```python
from build123d import *

# Parameters (mm, degrees)
SKETCH1_W           = 736.6
SKETCH1_H           = 381
BOSS_EXTRUDE1_DEPTH = 76.2
SKETCH2_W           = 50.8
SKETCH2_H           = 76.2
BOSS_EXTRUDE2_DEPTH = 254
SKETCH3_R           = 12.7
CUT_EXTRUDE1_DEPTH  = 503.413027299
SHELL1_T            = -2.54
SKETCH4_R           = 184.15
CUT_EXTRUDE2_DEPTH  = 2.54
SKETCH5_R           = 6.621401099
CUT_EXTRUDE3_DEPTH  = 1219.2


with BuildPart() as part:
    # Sketch1 → Boss-Extrude1 (new body)
    with BuildSketch(Plane(origin=(0, 0, 0), x_dir=(1, 0, 0), z_dir=(0, 1, 0))):
        Rectangle(SKETCH1_W, SKETCH1_H)
    extrude(amount=BOSS_EXTRUDE1_DEPTH)

    # Sketch2 → Boss-Extrude2 (add)
    with BuildSketch(Plane(origin=(0, 0, 0), x_dir=(-1, 0, 0), z_dir=(0, -1, 0))):
        with Locations((-317.5, 0)):
            Rectangle(SKETCH2_W, SKETCH2_H)
    extrude(amount=BOSS_EXTRUDE2_DEPTH)

    # Sketch3 → Cut-Extrude1 (cut, through all)
    with BuildSketch(Plane.XY.offset(38.1)):
        with Locations((317.5, -228.6)):
            Circle(SKETCH3_R)
    extrude(amount=-CUT_EXTRUDE1_DEPTH, mode=Mode.SUBTRACT)

    # Shell1
    shell1_openings = [part.faces().sort_by_distance(p)[0] for p in [
        (-368.3, 38.1, 0),
        (368.3, 38.1, 0),
    ]]
    offset(amount=SHELL1_T, openings=shell1_openings, kind=Kind.INTERSECTION)

    # Sketch4 → Cut-Extrude2 (cut)
    with BuildSketch(Plane(origin=(0, 76.2, 0), x_dir=(1, 0, 0), z_dir=(0, 1, 0))):
        with Locations(Location((-63.5, 0, 0), (0, 0, 270))):
            Circle(SKETCH4_R)
    extrude(amount=-CUT_EXTRUDE2_DEPTH, mode=Mode.SUBTRACT)

    # Sketch5 → Cut-Extrude3 (cut)
    with BuildSketch(Plane(origin=(0, 76.2, 0), x_dir=(1, 0, 0), z_dir=(0, 1, 0))):
        with Locations(Location((-63.5, 0, 0), (0, 0, 270))):
            Circle(SKETCH5_R)
    extrude(amount=-CUT_EXTRUDE3_DEPTH, mode=Mode.SUBTRACT)


solid = part.part
```
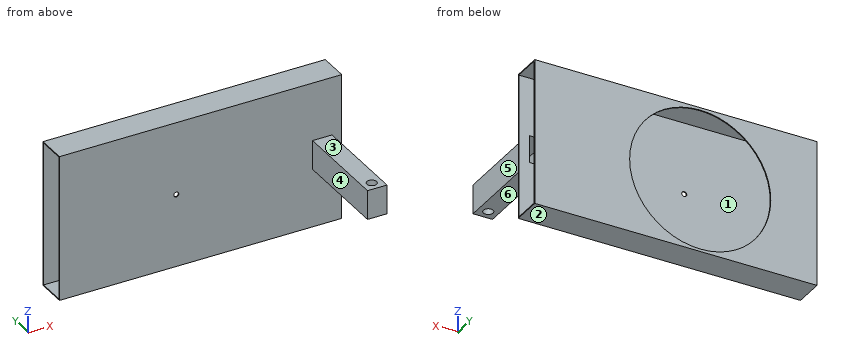
Geometry check sheet. Reference: the model listing, model coordinates, mm. Face numbers are marked on the shaded views. A direction names the side the tool comes from. Coordinates: 2 decimals unless noted, no trailing zeros. Order: outer loops, then holes, each group sorted by start corner. A loop starts at its lowest first (then second) coordinate and runs counter-clockwise, first axis right, second up. Notation, with made-up numbers: (82, -17.5) - (100, -17.5) arc R26 ccw to (100, 0.5) - close; hole circle Ø7 at (4, -2). An arc over 180 degrees is marked (long way). Answer in a Markdown table with one row per item. Add a question column.
1. Section check C-C (x = 168.5). Enter the section's corners in (y, z).
2. Access from +Z, -Z, +X, -X, +Y, -Y to the whole of each face (thin tool, end or side, straight path). Record for the marked faces 1, 2 and 3.
3. Section check B-B (x = 317.5). Enter the section's corners in (y, z), plus the area to 3 significant figures.
4. Material ranges on L1, parallel to X at y = 1, z = 0; L2, parallel to Y at x = 317, z = 21; L3, parallel to Y at x = -210.5, z = -165, recorded low to high. Write a range as [from, to].
5. Section check A-A (y = 13). Enter the section's corners in (x, z).
6. Section check D-D (y = -32.5). Enter the section's corners in (x, z).
7. Gauge pin test, flat ends, axial feed: pin 1 Ø1.5 at (x, z) = (136, 3.5) entering from -Y; pin 2 Ø23 at (x, y) = (307, -167) entering from +Z. Record the tip position at first contact, or that the pin passes through.
8. Draft check along X on the marked faces 4, 5 and 6. Enter one of: +X half, -X half, draft (parallel to the pull), parting line (faces both ways), or undercut.
Data:
| question | item | result |
|---|---|---|
| 1 | outline | (0, -190.5) - (76.2, -190.5) - (76.2, 190.5) - (0, 190.5) - close; hole (2.54, -187.96) - (73.66, -187.96) - (73.66, 187.96) - (2.54, 187.96) - close |
| 2 | face 1 | +X, -X |
| 2 | face 2 | -Z, +X, -X, +Y, -Y |
| 2 | face 3 | +Z, +X, -X, -Y |
| 3 | outline | (-254, -38.1) - (-241.3, -38.1) - (-241.3, 38.1) - (-254, 38.1) - close; (-215.9, -38.1) - (0, -38.1) - (0, -190.5) - (76.2, -190.5) - (76.2, 190.5) - (0, 190.5) - (0, 38.1) - (-215.9, 38.1) - close; hole (-251.46, -35.56) - (-243.84, -35.56) - (-243.84, 35.56) - (-251.46, 35.56) - close; hole (-213.36, -35.56) - (2.54, -35.56) - (2.54, -187.96) - (73.66, -187.96) - (73.66, 187.96) - (2.54, 187.96) - (2.54, 35.56) - (-213.36, 35.56) - close |
| 3 | area | 3,820 mm² |
| 4 | L1 | x = [-368.3, -70.12], [-56.88, 294.64], [340.36, 368.3] |
| 4 | L2 | y = [-254, -251.46], [-243.83, -241.29], [-215.91, -213.37], [73.66, 76.2] |
| 4 | L3 | y = [0, 2.54], [73.66, 76.2] |
| 5 | outline | (-368.3, -190.5) - (368.3, -190.5) - (368.3, -187.96) - (-368.3, -187.96) - close; (-368.3, 187.96) - (368.3, 187.96) - (368.3, 190.5) - (-368.3, 190.5) - close |
| 6 | outline | (292.1, -38.1) - (342.9, -38.1) - (342.9, 38.1) - (292.1, 38.1) - close; hole (294.64, -35.56) - (340.36, -35.56) - (340.36, 35.56) - (294.64, 35.56) - close |
| 7 | pin 1 | stops at y = 0 |
| 7 | pin 2 | stops at z = 38.1 |
| 8 | face 4 | -X half |
| 8 | face 5 | +X half |
| 8 | face 6 | draft |
